Could you check a few things on this model? Use its own coordinates, in mm. A direction names the side the tool comes from. Round coordinates to 2 decimals unless told otherwise and drop trailing zeros. Loops run counter-clockwise (first coordinate to the right, second up) from the corner with the lowest first, then second, coordinate; pieces in that order, holes last. Notation, with made-up numbers: (76, 80) - (95, 80) arc R25 ccw to (95, 101) - close; hole circle Ø2 at (14, -36.75). An arc over 180 degrees is marked (long way). Answer as CSV lines item,"result". Start each with the question number.
1) Suppose I cut it at A-A, the plane y = 21. Write out the boundary of the cut face in (x, z).
2) Suppose I cut it at D-D, the plane y = 32. Write out the boundary of the cut face in (x, z).
3) I'm going to push flat-ended pins straight in: pin 1 Ø8 at (x, y) = (19.5, 31) entering from -Z; pin 2 Ø4 at (x, z) = (-25, 97.75) entering from +Y; pin 3 Ø8 at (x, z) = (-1, 77.5) entering from -Y. Where does each tip first touch, or does it pass through?
4) Suppose I cut it at C-C, the plane x = 19.5. Write out the boundary of the cut face in (y, z).
5) Suppose I cut it at B-B, the plane z = 3. Write out the boundary of the cut face in (x, y).
6) We'd pull the mould along X, two halves only. Please class faces 1 (the face through (-13.45, 10.15, 60.89)), 2 (the face through (3.33, 38.7, -7.69)), 3 (the face through (-25, 7.5, 61)): pulls with the +X half, pulls with the -X half, needs draft (parallel to the pull), parting line crosses it, or undercut.
7) Which directions (+Z, -Z, +X, -X, +Y, -Y) give clear straight access to the entire face, cutting with the end or side of a thin tool? Please do faces 4 (the face through (13.549, 10.074, 60.886)), 5 (the face through (-23, 47, 95)), 6 (the face through (35, 32, 61)), 7 (the face through (0, 32, 123.5)), 8 (the face through (-15.188, 27.238, 60.886)).
8) Please list where these lines run through material, in increasing order: line 1 along Z through (x, y) = (-25, 48); line 2 along X through (y, z) = (49.75, 25.75); line 3 along X through (y, z) = (14, 87.5).
```python
from build123d import *

# Parameters (mm, degrees)
EXTRUDE_1_DEPTH        = 123.5
CHAMFER_1_SIZE         = 1
HOLE_WIZARD_M8_1_D     = 6.8
HOLE_WIZARD_M8_1_DEPTH = 15
HOLE_WIZARD_M8_1_TIP   = 2.042926105
SKETCH_5_R             = 5.961453201
EXTRUDE_2_DEPTH        = 15.6


with BuildPart() as part:
    # 草圖2 → 伸長1 (new body)
    with BuildSketch(Plane.XY):
        Polygon((-17, 7.5), (-35, 7.5), (-35, 55), (35, 55), (35, 7.5), (17, 7.5), (10, 12.721375014), (10, 16.129907798), (17, 23.129907798), (17, 25.4259063), (13.4259063, 29), (-13.4259063, 29), (-17, 25.4259063), (-17, 23.129907798), (-10, 16.129907798), (-10, 12.721375014), align=None)
    extrude(amount=EXTRUDE_1_DEPTH)

    # 導角1
    chamfer_1_edges = [part.edges().sort_by_distance(p)[0] for p in [
        (-35, 7.5, 61.75),
        (-35, 55, 61.75),
        (35, 55, 61.75),
        (35, 7.5, 61.75),
    ]]
    chamfer(chamfer_1_edges, length=CHAMFER_1_SIZE)

    # M8 螺紋孔1
    with Locations(Plane(origin=(0, 55, 0), x_dir=(-1, 0, 0), z_dir=(0, 1, 0))):
        with Locations((25, 97.75), (25, 25.75), (-25, 25.75), (-25, 97.75)):
            Hole(HOLE_WIZARD_M8_1_D / 2, depth=HOLE_WIZARD_M8_1_DEPTH)
            with Locations((0, 0, -(HOLE_WIZARD_M8_1_DEPTH + HOLE_WIZARD_M8_1_TIP / 2))):  # 118° drill point
                Cone(0, HOLE_WIZARD_M8_1_D / 2, HOLE_WIZARD_M8_1_TIP, mode=Mode.SUBTRACT)

    # 草圖5 → 伸長2 (add)
    with BuildSketch(Plane(origin=(0, 0, 0), x_dir=(-1, 0, 0), z_dir=(0, 0, -1))):
        with Locations((-2.037583141, 44.518465944)):
            Circle(SKETCH_5_R)
    extrude(amount=EXTRUDE_2_DEPTH)


solid = part.part
```
Filled sheet:
1,outline,"(-35, 0) - (-14.87, 0) - (-14.87, 123.5) - (-35, 123.5) - close; (14.87, 0) - (35, 0) - (35, 123.5) - (14.87, 123.5) - close"
2,outline,"(-35, 0) - (35, 0) - (35, 123.5) - (-35, 123.5) - close"
3,pin 1,"z = 0"
3,pin 2,"y = 39.16"
3,pin 3,"y = 29"
4,outline,"(7.5, 0) - (55, 0) - (55, 123.5) - (7.5, 123.5) - close"
5,outline,"(-35, 8.5) - (-34, 7.5) - (-17, 7.5) - (-10, 12.72) - (-10, 16.13) - (-17, 23.13) - (-17, 25.43) - (-13.43, 29) - (13.43, 29) - (17, 25.43) - (17, 23.13) - (10, 16.13) - (10, 12.72) - (17, 7.5) - (34, 7.5) - (35, 8.5) - (35, 54) - (34, 55) - (-34, 55) - (-35, 54) - close"
6,face 1,"undercut"
6,face 2,"parting line crosses it"
6,face 3,"needs draft"
7,face 4,"+Z, -Z, -Y"
7,face 5,"+Y"
7,face 6,"+Z, -Z, +X, +Y, -Y"
7,face 7,"+Z, +X, -X, +Y, -Y"
7,face 8,"+Z, -Z"
8,line 1,"0 to 22.35, 29.15 to 94.35, 101.15 to 123.5"
8,line 2,"-35 to -28.4, -21.6 to 21.6, 28.4 to 35"
8,line 3,"-35 to -10, 10 to 35"
